Verification items for the finished model (mm, model axes). A direction names the side the tool comes from. Coordinates: 2 decimals unless noted, no trailing zeros. Order: outer loops, then holes, each group sorted by start corner. A loop starts at its lowest first (then second) coordinate and runs counter-clockwise, first axis right, second up.
Q1. Set-up check for faces 1 (the flat face through (47, 12.5, 50)), 2 (the flat face through (76.455, 6, 66)), 3 (the flat face through (96, -12, 40.248)): record each of +Z, -Z, +X, -X, +Y, -Y from which the full face is reachable in a straight line by a thin tool's end or side.
Q2. Cross-section at B-B, the plane z = 52. Record the boundary of the cut face in (x, y), and give its area (3 significant figures).
Q3. Cross-section at A-A, the plane y = -10. Record the boundary of the cut face in (x, z), and give its area (3 significant figures).
Q4. Cross-section at C-C, the plane z = 22.5. Record the boundary of the cut face in (x, y), and give its area (3 significant figures).
Q5. Draft check along X on faces 4 (the flat face through (97, -12, 74.602)), 5 (the flat face through (76.455, -12, 51)), 6 (the flat face through (38.151, -6, 30)). Enter one of: pulls with the +X half, pulls with the -X half, needs draft (parallel to the pull), parting line crosses it, or undercut.
Q6. Depth check by flat-ended pin: P1, Ø7.5, axis at x = 94, y = -8, coming from the -Z side; P2, Ø6, axis at y = -12, z = 31.5, coming from the +X side; P3, Ø11, axis at y = -12.5, z = 23, coming from the -X side. Enter the tip coordinate at first touch or a pass-through.
Q7. Cross-section at D-D, the plane x = 86.5. Record the boundary of the cut face in (y, z).
Q8. Thickness scan on line 1 (X direction, y = 4, z = 43); line 2 (Z direction, x = 37.5, y = -19); line 3 (X direction, y = -9, z = -0.5). Record the ranges inside material, lowest first.
from build123d import *

# Parameters (mm, degrees)
F1_DEPTH = 20
F2_DEPTH = 12.5
F3_DEPTH = 25
F4_DEPTH = 25


with BuildPart() as f1:
    # F0 (on Front) → F1 (new body, symmetric)
    with BuildSketch(Plane.XZ):
        Polygon((48.5, -11.5), (48.5, 11.5), (38.151402, 11.5), (-48.5, 11.5), (-48.5, -11.5), align=None)
    extrude(amount=F1_DEPTH, both=True)

    # F0 (on Front) → F2 (join, symmetric)
    with BuildSketch(Plane.XZ):
        with BuildLine():
            Line((38.151402, 11.5), (48.5, 11.5))
            Line((48.5, 11.5), (48.5, 48.114586))
            ThreePointArc((48.5, 48.114586), (52.140113, 56.902597), (60.928124, 60.54271))
            Line((60.928124, 60.54271), (76.454861, 60.54271))
            Line((76.454861, 60.54271), (76.454861, 70.891308))
            Line((76.454861, 70.891308), (64.704314, 70.891308))
            add(Edge.make_bspline(
                [(57.274692, 70.59639), (59.883301, 70.756612), (62.369155, 70.854308), (64.704314, 70.891308)],
                knots=[119.890309, 119.890309, 119.890309, 119.890309, 127.668117, 127.668117, 127.668117, 127.668117], degree=3))
            ThreePointArc((57.274692, 70.59639), (43.578884, 62.872057), (38.151402, 48.114586))
            Line((38.151402, 48.114586), (38.151402, 11.5))
        make_face()
    extrude(amount=F2_DEPTH, both=True)

    # F0 (on Front) → F3 (join)
    with BuildSketch(Plane.XZ):
        Polygon((48.5, -11.5), (48.5, 11.5), (38.151402, 11.5), (-48.5, 11.5), (-48.5, -11.5), align=None)
        with BuildLine():
            Line((38.151402, 11.5), (48.5, 11.5))
            Line((48.5, 11.5), (48.5, 48.114586))
            ThreePointArc((48.5, 48.114586), (52.140113, 56.902597), (60.928124, 60.54271))
            Line((60.928124, 60.54271), (76.454861, 60.54271))
            Line((76.454861, 60.54271), (76.454861, 70.891308))
            Line((76.454861, 70.891308), (64.704314, 70.891308))
            add(Edge.make_bspline(
                [(57.274692, 70.59639), (59.883301, 70.756612), (62.369155, 70.854308), (64.704314, 70.891308)],
                knots=[119.890309, 119.890309, 119.890309, 119.890309, 127.668117, 127.668117, 127.668117, 127.668117], degree=3))
            ThreePointArc((57.274692, 70.59639), (43.578884, 62.872057), (38.151402, 48.114586))
            Line((38.151402, 48.114586), (38.151402, 11.5))
        make_face()
        with BuildLine():
            ThreePointArc((60.928124, 70.891308), (59.095466, 70.817459), (57.274692, 70.59639))
            add(Edge.make_bspline(
                [(57.274692, 70.59639), (59.883301, 70.756612), (62.369155, 70.854308), (64.704314, 70.891308)],
                knots=[119.890309, 119.890309, 119.890309, 119.890309, 127.668117, 127.668117, 127.668117, 127.668117], degree=3))
            Line((64.704314, 70.891308), (60.928124, 70.891308))
        make_face()
        Polygon((76.454861, 70.891308), (76.454861, 60.54271), (76.454861, 40.248264), (116.871528, 40.248264), (116.871528, 74.602442), (76.454861, 74.602442), align=None)
    extrude(amount=F3_DEPTH)

    # F0 (on Front) → F4 (join)
    with BuildSketch(Plane.XZ):
        Polygon((48.5, -11.5), (48.5, 11.5), (38.151402, 11.5), (-48.5, 11.5), (-48.5, -11.5), align=None)
        with BuildLine():
            Line((38.151402, 11.5), (48.5, 11.5))
            Line((48.5, 11.5), (48.5, 48.114586))
            ThreePointArc((48.5, 48.114586), (52.140113, 56.902597), (60.928124, 60.54271))
            Line((60.928124, 60.54271), (76.454861, 60.54271))
            Line((76.454861, 60.54271), (76.454861, 70.891308))
            Line((76.454861, 70.891308), (64.704314, 70.891308))
            add(Edge.make_bspline(
                [(57.274692, 70.59639), (59.883301, 70.756612), (62.369155, 70.854308), (64.704314, 70.891308)],
                knots=[119.890309, 119.890309, 119.890309, 119.890309, 127.668117, 127.668117, 127.668117, 127.668117], degree=3))
            ThreePointArc((57.274692, 70.59639), (43.578884, 62.872057), (38.151402, 48.114586))
            Line((38.151402, 48.114586), (38.151402, 11.5))
        make_face()
        with BuildLine():
            ThreePointArc((60.928124, 70.891308), (59.095466, 70.817459), (57.274692, 70.59639))
            add(Edge.make_bspline(
                [(57.274692, 70.59639), (59.883301, 70.756612), (62.369155, 70.854308), (64.704314, 70.891308)],
                knots=[119.890309, 119.890309, 119.890309, 119.890309, 127.668117, 127.668117, 127.668117, 127.668117], degree=3))
            Line((64.704314, 70.891308), (60.928124, 70.891308))
        make_face()
        Polygon((76.454861, 70.891308), (76.454861, 60.54271), (76.454861, 40.248264), (116.871528, 40.248264), (116.871528, 74.602442), (76.454861, 74.602442), align=None)
    extrude(amount=F4_DEPTH)


solid = f1.part
Check values:
1. face 1: +Z, +X, -X, +Y
1. face 2: +Z, -Z, +X, +Y
1. face 3: -Z, +X, +Y, -Y
2. outline: (38.49, -25) - (49.12, -25) - (49.12, 12.5) - (38.49, 12.5) - close; (76.45, -25) - (116.87, -25) - (116.87, 0) - (76.45, 0) - close
2. area: 1,410 mm2
3. outline: (-48.5, -11.5) - (48.5, -11.5) - (48.5, 48.11) arc R12.43 cw to (60.93, 60.54) - (76.45, 60.54) - (76.45, 40.25) - (116.87, 40.25) - (116.87, 74.6) - (76.45, 74.6) - (76.45, 70.89) - (60.93, 70.89) arc R22.78 ccw to (57.27, 70.6) arc R22.78 ccw to (38.15, 48.11) - (38.15, 11.5) - (-48.5, 11.5) - close
3. area: 4,450 mm2
4. outline: (38.15, -25) - (48.5, -25) - (48.5, 12.5) - (38.15, 12.5) - close
4. area: 388 mm2
5. face 4: needs draft
5. face 5: undercut
5. face 6: pulls with the -X half
6. P1: stops at z = 40.25
6. P2: stops at x = 48.5
6. P3: stops at x = 38.15
7. outline: (-25, 40.25) - (0, 40.25) - (0, 74.6) - (-25, 74.6) - close
8. line 1: x = 38.15 to 48.5
8. line 2: z = -11.5 to 11.5
8. line 3: x = -48.5 to 48.5
